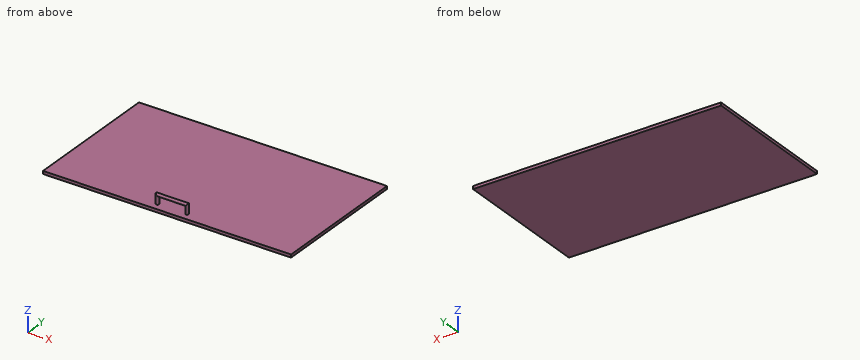
from build123d import *

# Parameters (mm, degrees)
SKETCH1_W           = 838.48
SKETCH1_H           = 471.91
BOSS_EXTRUDE1_DEPTH = 10
SKETCH2_R           = 5


with BuildPart() as part:
    # Sketch1 → Boss-Extrude1 (new body)
    with BuildSketch(Plane.XY):
        Rectangle(SKETCH1_W, SKETCH1_H)
    extrude(amount=BOSS_EXTRUDE1_DEPTH)

    # Sweep3: sweep along a curve in space
    with BuildLine() as sweep3_path:
        Line((-50, -210, 10), (-50, -210, 40))
        Line((50, -210, 40), (-50, -210, 40))
        Line((50, -210, 10), (50, -210, 40))
    # Sketch2 → Sweep3 (sweep)
    with BuildSketch(Plane.XY.offset(10)):
        with Locations((50, -210)):
            Circle(SKETCH2_R)
    sweep(path=sweep3_path.line, transition=Transition.RIGHT)


solid = part.part
The listing builds one solid part. Answer for the finished solid, in the listing's coordinates (mm). Give positions to 0.01 mm unless a question says otherwise; leave off trailing zeros. Loops run counter-clockwise (first coordinate to the right, second up) from the corner with the lowest first, then second, coordinate; pieces in that order, holes last. Notation, with made-up numbers: (45.5, 48) - (86.5, 48) arc R14 ccw to (86.5, 63) - close; hole circle Ø11 at (-39, 31). An arc over 180 degrees is marked (long way). Use one line per item in the form item = value.
1. Given pin 1 Ø5 at (x, y) = (60, -64.5) entering from +Z, flat-ended and moving along its own axis, determine where the tip first touches the part or whether it passes through.
Calculated:
pin_1 = 10
2. Section A-A on x = -15.5 is taken. Give the vertices of the cut face in (y, z) (3 decimals).
Calculated:
outline = (-235.955, 0) - (235.955, 0) - (235.955, 10) - (-235.955, 10) - close; circle Ø10 at (-210, 40)
3. Find the intervals of material crossed by line 1 along Z through (x, y) = (-168, 49.5), in increasing order. Write a range as [from, to].
Calculated:
line_1 = [0, 10]
4. Section B-B on z = 27.5 is taken. Give the vertices of the cut face in (x, y), then the cut area to 3 significant figures.
Calculated:
outline = circle Ø10 at (-50, -210); circle Ø10 at (50, -210)
area = 157 mm^2
5. Section D-D on x = -290 is taken. Give the vertices of the cut face in (y, z) (3 decimals), then the cut area to 3 significant figures.
Calculated:
outline = (-235.955, 0) - (235.955, 0) - (235.955, 10) - (-235.955, 10) - close
area = 4,720 mm^2
6. Section C-C on y = 42.5 is taken. Give the vertices of the cut face in (x, z), then the cut area to 3 significant figures.
Calculated:
outline = (-419.24, 0) - (419.24, 0) - (419.24, 10) - (-419.24, 10) - close
area = 8,380 mm^2
